The listing builds one solid part. Answer for the finished solid, in the listing's coordinates (mm). A direction names the side the tool comes from. Coordinates: 2 decimals unless noted, no trailing zeros. Order: outer loops, then holes, each group sorted by start corner. A loop starts at its lowest first (then second) coordinate and runs counter-clockwise, first axis right, second up. Notation, with made-up numbers: (14.25, 88) -> (47.25, 88) arc R26 cw to (47.25, 126) -> close; hole circle Ø8 at (7.5, -2.75). An arc over 180 degrees is marked (long way). Write item = value, one per line.
from build123d import *

# Parameters (mm, degrees)
BOSS_EXTRUDE2_DEPTH = 10


with BuildPart() as part:
    # Sketch1 → Boss-Extrude2 (new body)
    with BuildSketch(Plane.XY):
        with BuildLine():
            Line((0, 0), (2, 0))
            Line((2, 0), (2, -10.101020514))
            ThreePointArc((2, -10.101020514), (0.647580015, -13.895753707), (-2.8, -15.979795897))
            ThreePointArc((-2.8, -15.979795897), (-5.098386677, -17.369157357), (-6, -19.898979486))
            Line((-6, -19.898979486), (-6, -30))
            Line((-6, -30), (-8, -30))
            Line((-8, -30), (-8, -19.898979486))
            ThreePointArc((-8, -19.898979486), (-6.647580015, -16.104246293), (-3.2, -14.020204103))
            ThreePointArc((-3.2, -14.020204103), (-0.901613323, -12.630842643), (0, -10.101020514))
            Line((0, -10.101020514), (0, 0))
        make_face()
    extrude(amount=-BOSS_EXTRUDE2_DEPTH)


solid = part.part
Q1. A tool of negligible diameter and unlimited length cuts with its end or side. For faces 1 (the face through (-6, -25, -5)), 2 (the face through (-7, -30, -5)), 3 (the face through (0, -5, -5)), from which of +Z, -Z, +X, -X, +Y, -Y can it reach the whole face along a straight path? Write none if from no direction.
The answers:
face_1 = +Z, -Z, +X, -Y
face_2 = +Z, -Z, +X, -X, -Y
face_3 = +Z, -Z, -X, +Y
Q2. Each of these flat-tipped pins is pushed along its axis until it touches: pin 1 Ø6 at (x, z) = (-5.5, -9) entering from +Y; pin 2 Ø3 at (x, z) = (-1, -7) entering from +Y; pin 3 Ø1 at (y, z) = (-19.5, -4) entering from +X; pin 4 Ø3 at (y, z) = (-16, -2) entering from +X. Where does it stop, or does it pass through?
The answers:
pin_1 = -13.81
pin_2 = 0
pin_3 = -5.9
pin_4 = 0.08
Q3. Section A-A, the plane z = -1.5 is taken. Give the vertices of the cut face in (x, y).
The answers:
outline = (-8, -30) -> (-6, -30) -> (-6, -19.9) arc R4 cw to (-2.8, -15.98) arc R6 ccw to (2, -10.1) -> (2, 0) -> (0, 0) -> (0, -10.1) arc R4 cw to (-3.2, -14.02) arc R6 ccw to (-8, -19.9) -> close
Q4. Section B-B, the plane y = -28 is taken. Give the vertices of the cut face in (x, z).
The answers:
outline = (-8, -10) -> (-6, -10) -> (-6, 0) -> (-8, 0) -> close
Q5. Find the intervals of material crossed by line 1 along X through (y, z) = (-5.25, -5); line 2 along X through (y, z) = (-23.75, -8); line 3 along Y through (x, z) = (-3.75, -1.5), in increasing order.
The answers:
line_1 = 0 to 2
line_2 = -8 to -6
line_3 = -16.3 to -14.16
Q6. Section C-C, the plane x = -5.25 is taken. Give the vertices of the cut face in (y, z), plus the area to 3 significant figures.
The answers:
outline = (-17.57, -10) -> (-14.86, -10) -> (-14.86, 0) -> (-17.57, 0) -> close
area = 27.1 mm2
